from build123d import *

# Parameters (mm, degrees)
SKETCH2_W           = 88.9
SKETCH2_H           = 41.91
BOSS_EXTRUDE1_DEPTH = 2.54
SKETCH3_R           = 1.651
CUT_EXTRUDE2_DEPTH  = 50.207378766
SKETCH4_W           = 76.2
SKETCH4_H           = 29.21
BOSS_EXTRUDE2_DEPTH = 22.86


with BuildPart() as part:
    # Sketch2 → Boss-Extrude1 (new body)
    with BuildSketch(Plane(origin=(0, 0, 0), x_dir=(1, 0, 0), z_dir=(0, 1, 0))):
        Rectangle(SKETCH2_W, SKETCH2_H)
    extrude(amount=BOSS_EXTRUDE1_DEPTH)

    # Sketch3 → Cut-Extrude2 (cut, through all)
    with BuildSketch(Plane(origin=(0, 0, 0), x_dir=(1, 0, 0), z_dir=(0, 1, 0))):
        with Locations(Location((-40.64, 17.145, 0), (0, 0, 270))):
            Circle(SKETCH3_R)
        with Locations(Location((40.64, 17.145, 0), (0, 0, 270))):
            Circle(SKETCH3_R)
        with Locations(Location((40.64, -17.145, 0), (0, 0, 270))):
            Circle(SKETCH3_R)
        with Locations(Location((-40.64, -17.145, 0), (0, 0, 270))):
            Circle(SKETCH3_R)
    extrude(amount=CUT_EXTRUDE2_DEPTH, mode=Mode.SUBTRACT)

    # Sketch4 → Boss-Extrude2 (add)
    with BuildSketch(Plane(origin=(0, 2.54, 0), x_dir=(1, 0, 0), z_dir=(0, 1, 0))):
        Rectangle(SKETCH4_W, SKETCH4_H)
    extrude(amount=BOSS_EXTRUDE2_DEPTH)


solid = part.part
For this review, take the finished solid that the model builds, in its own axes (mm). A direction names the side the tool comes from. Round coordinates to 2 decimals unless told otherwise and drop trailing zeros. Write each loop counter-clockwise with the first axis right and the second up, starting at its lowest first coordinate (ties: lowest second). Pieces come first, ordered by that corner, then holes. Notation, with made-up numbers: M 22,24.5 L 64,24.5 A23 ccw 64,55.5 Z; hole C -38.5,64 d1. An arc over 180 degrees is marked long. Write item = value, one per line. Start each with the question number.
(1) We need section B-B (z = 4). Give the boundary of the cut face in (x, y).
(2) We need section D-D (y = 17.25). Give the boundary of the cut face in (x, z) (3 decimals), then the cut area to 3 significant figures.
(3) We need section A-A (x = 40.64). Give the boundary of the cut face in (y, z) (3 decimals), then the cut area to 3 significant figures.
(4) For line 1 along Z through (x, y) = (-40.64, 1.6) (3 decimals); line 2 along X through (y, z) = (6.75, 13); line 3 along Z through (x, y) = (31, 7) (3 decimals), list the stretches that pass through material, from the lowest coordinate up.
(5) The part is to be moulded in two halves that separate along X. For faces 4 (the face through (42.277, 1.252, -17.36)), 5 (the face through (38.1, 14, 0)), 6 (the face through (-1, 2.54, -19)), say which applies: +X half, -X half, draft (parallel to the pull), parting line (faces both ways), or undercut.
(6) We need section C-C (x = -9). Give the boundary of the cut face in (y, z) (3 decimals).
(7) Clearance check with flat-ended pins moving along their axes: pin 1 Ø6 at (y, z) = (11, 16.5) entering from +X; pin 2 Ø11.5 at (x, y) = (-6, 14.5) entering from -Z (3 decimals); pin 3 Ø4 at (x, z) = (-40.64, 17.145) entering from +Y; pin 4 Ø2 at (y, z) = (7.5, -16.5) entering from -X. State where each tip first meets the part, or that it passes through.
(8) For faces 1 (the face through (-1, 14, -14.605)), 2 (the face through (-38.1, 14, 0)), 3 (the face through (-1, 14, 14.605)), list the 3-axis set-ups (+Z, -Z, +X, -X, +Y, -Y) from which the entire face can be reached by the end or side of a thin tool; tool diameter is ignored.
Results found:
q1.outline = M -44.45,0 L 44.45,0 L 44.45,2.54 L 38.1,2.54 L 38.1,25.4 L -38.1,25.4 L -38.1,2.54 L -44.45,2.54 Z
q2.outline = M -38.1,-14.605 L 38.1,-14.605 L 38.1,14.605 L -38.1,14.605 Z
q2.area = 2,230 mm²
q3.outline = M 0,-20.955 L 2.54,-20.955 L 2.54,-18.796 L 0,-18.796 Z; M 0,-15.494 L 2.54,-15.494 L 2.54,15.494 L 0,15.494 Z; M 0,18.796 L 2.54,18.796 L 2.54,20.955 L 0,20.955 Z
q3.area = 89.7 mm²
q4.line_1 = -20.955 to -18.796, -15.494 to 15.494, 18.796 to 20.955
q4.line_2 = -38.1 to 38.1
q4.line_3 = -14.605 to 14.605
q5.face_4 = undercut
q5.face_5 = +X half
q5.face_6 = draft
q6.outline = M 0,-20.955 L 2.54,-20.955 L 2.54,-14.605 L 25.4,-14.605 L 25.4,14.605 L 2.54,14.605 L 2.54,20.955 L 0,20.955 Z
q7.pin_1 = 38.1
q7.pin_2 = -14.605
q7.pin_3 = 2.54
q7.pin_4 = through
q8.face_1 = -Z, +X, -X, +Y
q8.face_2 = +Z, -Z, -X, +Y
q8.face_3 = +Z, +X, -X, +Y
